from build123d import *

# Parameters (mm, degrees)
BOSS_EXTRUDE1_DEPTH = 32.5
SKETCH4_R           = 0.5
BOSS_EXTRUDE2_DEPTH = 1


with BuildPart() as part:
    # Sketch2 → Boss-Extrude1 (new body)
    with BuildSketch(Plane.XY):
        with BuildLine():
            Line((0.25, 0), (2.83, 0))
            ThreePointArc((2.83, 0), (3.006776695, 0.073223305), (3.08, 0.25))
            Line((3.08, 0.25), (3.08, 2.83))
            ThreePointArc((3.08, 2.83), (3.006776695, 3.006776695), (2.83, 3.08))
            Line((2.83, 3.08), (0.25, 3.08))
            ThreePointArc((0.25, 3.08), (0.073223305, 3.006776695), (0, 2.83))
            Line((0, 2.83), (0, 0.25))
            ThreePointArc((0, 0.25), (0.073223305, 0.073223305), (0.25, 0))
        make_face()
    extrude(amount=BOSS_EXTRUDE1_DEPTH)

    # Sketch4 → Boss-Extrude2 (add)
    with BuildSketch(Plane(origin=(0, 0, 0), x_dir=(-1, 0, 0), z_dir=(0, 0, -1))):
        with Locations(Location((-1.54, 1.54, 0), (0, 0, 180))):
            Circle(SKETCH4_R)
    extrude(amount=BOSS_EXTRUDE2_DEPTH)


solid = part.part
Could you check a few things on this model? Use its own coordinates, in mm. A direction names the side the tool comes from. Coordinates: 2 decimals unless noted, no trailing zeros. Loops run counter-clockwise (first coordinate to the right, second up) from the corner with the lowest first, then second, coordinate; pieces in that order, holes last.
1. Imagine slicing it at A-A (y = 1.54). Please give me the cut outline in (x, z), and give its area (3 significant figures).
2. I need wall thicknesses on L1, parallel to Z at x = 1.95, y = 0.2. Which ranges of the line are inside material? Lowest first, please.
3. For faces 1 (the face through (1.5, 1.5, -1)), 2 (the face through (1, 2, 0)), which set-ups out of +Z, -Z, +X, -X, +Y, -Y let a thin tool reach every point of the face, with its end or its side?
Computed values:
1. outline: (0, 0) - (1.04, 0) - (1.04, -1) - (2.04, -1) - (2.04, 0) - (3.08, 0) - (3.08, 32.5) - (0, 32.5) - close
1. area: 101 mm2
2. L1: z = 0 to 32.5
3. face 1: -Z, +X, -X, +Y, -Y
3. face 2: -Z
